```python
from build123d import *

# Parameters (mm, degrees)
BOX_W                  = 7.071
BOX_H                  = 20
BOX_DEPTH              = 7.071
BOX_PITCH_ANGLE        = 45
BOX_PLACEMENT_ANGLE    = -11
BOX001_W               = 10
BOX001_H               = 20
BOX001_DEPTH           = 10
BOX001_PLACEMENT_ANGLE = 349


with BuildPart() as cub:
    # Box → Box (new body)
    with BuildSketch(Plane.XY):
        with Locations((3.5355, 10)):
            Rectangle(BOX_W, BOX_H)
    extrude(amount=BOX_DEPTH)


with BuildPart() as cub_1:
    # Box pitch: moved
    add(cub.part.rotate(Axis((0, 0, 0), (0, 1, 0)), BOX_PITCH_ANGLE))


with BuildPart() as cub_2:
    # Box placement: moved
    add(cub_1.part.moved(Location((-6.816226, -8.862227, 10))).rotate(Axis((-6.816226, -8.862227, 10), (0, 0, 1)), BOX_PLACEMENT_ANGLE))


with BuildPart() as fusion:
    # Box001 → Box001 (new body)
    with BuildSketch(Plane.XY):
        with Locations((5, 10)):
            Rectangle(BOX001_W, BOX001_H)
    extrude(amount=BOX001_DEPTH)


with BuildPart() as fusion_1:
    # Box001 placement: moved
    add(fusion.part.moved(Location((-6.816226, -8.862227, 0))).rotate(Axis((-6.816226, -8.862227, 0), (0, 0, 1)), BOX001_PLACEMENT_ANGLE))

    # Fusion: union Cub
    add(cub_2.part)


solid = fusion_1.part
```
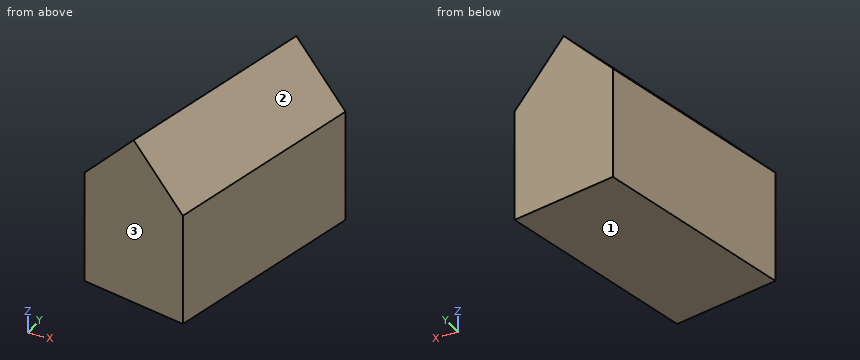
The listing builds one solid part. Answer for the finished solid, in the listing's coordinates (mm). Face numbers are marked on the shaded views. Give positions to 0.01 mm unless a question says otherwise; leave off trailing zeros. Order: outer loops, then holes, each group sorted by start corner. A loop starts at its lowest first (then second) coordinate and runs counter-clockwise, first axis right, second up.
1) Given P1, Ø4, axis at y = 1, z = 7, coming from the -X side; P2, Ø1, axis at y = 8.5, z = 11.5, coming from the +X side; P3, Ø3, axis at y = -4, z = 9, coming from the +X side, each flat-ended and moving along its own axis, determine where each tip first touches the part or whether it passes through.
Reported:
P1: stops at x = -5.29
P2: stops at x = 5.74
P3: stops at x = 4.61
2) Consider line 1 along X through (y, z) = (5, 4.75); line 2 along X through (y, z) = (5.75, 13.75); line 3 along Y through (x, z) = (-1.25, 8.25). Determine where each line is inside the solid, lowest interval first.
Reported:
line 1: x = -4.12 to 6.07
line 2: x = -0.16 to 2.39
line 3: y = -9.94 to 10.43
3) Find section D-D on z = 12.5. Write down the section's boundary in (x, y).
Reported:
outline: (-4.36, -9.34) - (0.55, -10.29) - (4.36, 9.34) - (-0.55, 10.29) - close
4) Find section A-A on z = 3. Write down the section's boundary in (x, y), then the cut area to 3 significant figures.
Reported:
outline: (-6.82, -8.86) - (3, -10.77) - (6.82, 8.86) - (-3, 10.77) - close
area: 200 mm2
5) Determine the mould class of the marked faces 1, 2 and 3 for opening direction Z: pulls with the +Z half, pulls with the -Z half, needs draft (parallel to the pull), parting line crosses it, or undercut.
Reported:
face 1: pulls with the -Z half
face 2: pulls with the +Z half
face 3: needs draft
6) Find section B-B on x = 0. Write down the section's boundary in (y, z), then the cut area to 3 significant figures.
Reported:
outline: (-10.19, 0) - (10.19, 0) - (10.19, 13.06) - (0, 15) - (-10.19, 13.06) - close
area: 286 mm2
